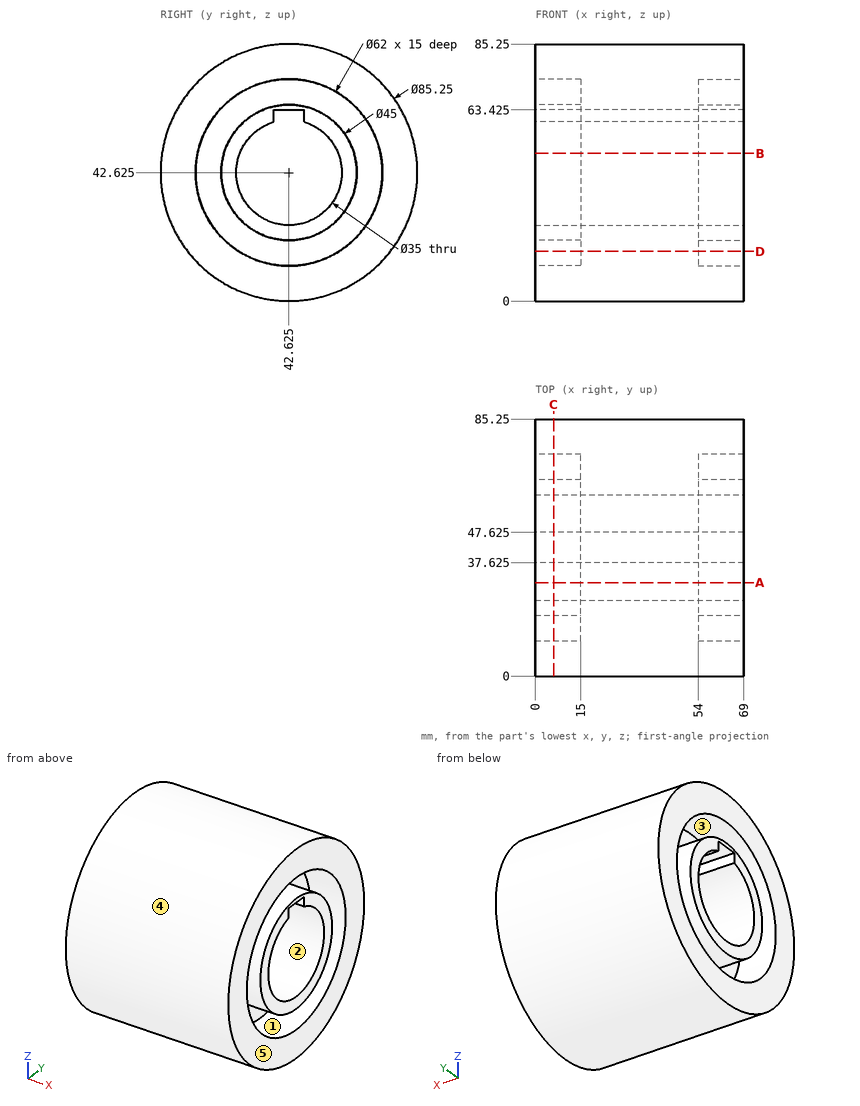
Geometry check sheet. Reference: drawing and pictorial views, mm from the part's lowest x, y, z. A direction names the side the tool comes from. Coordinates: 2 decimals unless noted, no trailing zeros. Order: outer loops, then holes, each group sorted by start corner. A loop starts at its lowest first (then second) coordinate and runs counter-clockwise, first axis right, second up.
Item 1: Section check A-A (y = 31). Enter the section's corners in (x, z).
Item 2: Section check D-D (z = 16.5). Enter the section's corners in (x, y).
Item 3: Section check C-C (x = 6). Count the separate pieces of the cut face and the enclosed holes in it, plus the area to 3 significant figures.
Item 4: Tool access check on the marked faces 1 and 2. Record the directions out of +Z, -Z, +X, -X, +Y, -Y that give a thin tool (end or side, any length) a straight path to the whole face; none if there is none.
Item 5: Scan lines: line 1 along Y through (x, z) = (58, 43.5); line 2 along Z through (x, y) = (55.5, 54.5); line 3 along Z through (x, y) = (64, 28). Record each from-to range of solid material in increasing order.
Item 6: Mould release check, pull along Z, two halves, no side actions. Record for the marked faces 3, 4 and 5: released by +Z, released by -Z, zero draft, split by the parting line, or undercut.
Item 7: Depth check by flat-ended pin: pin 1 (4.5 mm diameter, centred on x = 19, z = 60.5, fed in from +Y); pin 2 (2 mm diameter, centred on y = 62, z = 23.5, fed in from -X); pin 3 (1.5 mm diameter, centred on x = 20.5, y = 31.5, fed in from +Z). Enter the tip coordinate at first touch or a pass-through.
Item 8: Section check B-B (z = 49). Enter the section's corners in (x, y).
Check sheet entries:
1. outline: (0, 1.62) - (69, 1.62) - (69, 13.89) - (54, 13.89) - (54, 23.36) - (69, 23.36) - (69, 29.54) - (0, 29.54) - (0, 23.36) - (15, 23.36) - (15, 13.89) - (0, 13.89) - close; (0, 55.71) - (69, 55.71) - (69, 61.89) - (54, 61.89) - (54, 71.36) - (69, 71.36) - (69, 83.63) - (0, 83.63) - (0, 71.36) - (15, 71.36) - (15, 61.89) - (0, 61.89) - close
2. outline: (0, 8.94) - (69, 8.94) - (69, 25.94) - (54, 25.94) - (54, 59.31) - (69, 59.31) - (69, 76.31) - (0, 76.31) - (0, 59.31) - (15, 59.31) - (15, 25.94) - (0, 25.94) - close
3. separate pieces: 2
3. enclosed holes: 2
3. area: 3,280 mm2
4. face 1: +X
4. face 2: +X, -X
5. line 1: y = 0.01 to 11.64, 20.14 to 25.15, 60.1 to 65.11, 73.61 to 85.24
5. line 2: z = 1.69 to 13.99, 23.51 to 29.77, 55.48 to 61.74, 71.26 to 83.56
5. line 3: z = 2.59 to 15.29, 25.53 to 33.01, 52.24 to 59.72, 69.96 to 82.66
6. face 3: undercut
6. face 4: split by the parting line
6. face 5: zero draft
7. pin 1: stops at y = 82.28
7. pin 2: stops at x = 15
7. pin 3: stops at z = 83.97
8. outline: (0, 0.48) - (69, 0.48) - (69, 12.29) - (54, 12.29) - (54, 21.05) - (69, 21.05) - (69, 26.33) - (0, 26.33) - (0, 21.05) - (15, 21.05) - (15, 12.29) - (0, 12.29) - close; (0, 58.92) - (69, 58.92) - (69, 64.2) - (54, 64.2) - (54, 72.96) - (69, 72.96) - (69, 84.77) - (0, 84.77) - (0, 72.96) - (15, 72.96) - (15, 64.2) - (0, 64.2) - close
